Geometry: final body of the model. Coordinates: model frame, mm. Face numbers are marked on the shaded views. A direction names the side the tool comes from. Coordinates: 2 decimals unless noted, no trailing zeros. Order: outer loops, then holes, each group sorted by start corner. A loop starts at its lowest first (then second) coordinate and runs counter-clockwise, first axis right, second up. Notation, with made-up numbers: M -38.75,-17 L -0.75,-17 A25 ccw -0.75,5 Z; hole C 19,-24.5 d10. An arc over 180 degrees is marked long. Use CSV: the item, a comma, the result in double quotes. Start each with the question number.
Q1. Access query for the marked faces 4 and 5. Directions: +Z, -Z, +X, -X, +Y, -Y. A direction counts if a zero-diameter tool reaches every point of the face in a straight line with its end or side. Return the directions, or none.
Q2. Section query B-B, the plane x = 0. Output: boundary loops of the cut face in (y, z).
Q3. Section query A-A, the plane x = 28.5. Output: boundary loops of the cut face in (y, z).
Q4. First-contact query: P1, Ø12.5, axis at x = 10, z = 3, coming from the -Y side; P2, Ø12.5, axis at x = 0, z = 0, coming from the -Y side; P3, Ø1, axis at y = 7, z = 6.5, coming from the -X side; P4, Ø5, axis at x = 0, z = 0, coming from the -Y side. Flat tips, straight axial feed; report the tip coordinate or a pass-through.
Q5. Ray query, probe 1 along Y at (x, z) = (9, -11.25); probe 2 along X at (y, z) = (-23.35, 0); probe 3 along Z at (x, y) = (0, -21.3). Return the intervals inside material, ascending.
Q6. Mould query, pull axis Y, two halves, no side actions, for the marked faces 1, 2 and 3. Classes: +Y half, -Y half, draft (parallel to the pull), parting line (faces both ways), or undercut.
Q7. Section query C-C, the plane z = 6.5. Output: boundary loops of the cut face in (x, y), and give its area (3 significant figures).
Q8. Section query D-D, the plane x = 46. Output: boundary loops of the cut face in (y, z), and give its area (3 significant figures).
from build123d import *

# Parameters (mm, degrees)
CYLINDER018_R          = 4.1
CYLINDER018_DEPTH      = 10
CYLINDER018_ROLL_ANGLE = 90
CYLINDER016_R          = 10.55
CYLINDER016_DEPTH      = 10
CYLINDER016_ROLL_ANGLE = 90
PAD005_DEPTH           = 25
FILLET008_R            = 12.4


with BuildPart() as cilindro018:
    # Cylinder018 → Cylinder018 (new body)
    with BuildSketch(Plane.XY):
        Circle(CYLINDER018_R)
    extrude(amount=CYLINDER018_DEPTH)


with BuildPart() as cilindro018_1:
    # Cylinder018 roll: moved
    add(cilindro018.part.rotate(Axis((0, 0, 0), (1, 0, 0)), CYLINDER018_ROLL_ANGLE))


with BuildPart() as cilindro018_2:
    # Cylinder018 placement: moved
    add(cilindro018_1.part.moved(Location((0, -14, 0))))


with BuildPart() as obj1:
    # Cylinder016 → Cylinder016 (new body)
    with BuildSketch(Plane.XY):
        Circle(CYLINDER016_R)
    extrude(amount=CYLINDER016_DEPTH)


with BuildPart() as obj1_1:
    # Cylinder016 roll: moved
    add(obj1.part.rotate(Axis((0, 0, 0), (1, 0, 0)), CYLINDER016_ROLL_ANGLE))


with BuildPart() as obj1_2:
    # Cylinder016 placement: moved
    add(obj1_1.part.moved(Location((0, -22.5, 0))))

    # Fusion002: union Cilindro018
    add(cilindro018_2.part)


with BuildPart() as cut023004:
    # Sketch005 → Pad005 (new body)
    with BuildSketch(Plane(origin=(0, 0, 12.5), x_dir=(-1, 0, 0), z_dir=(0, 0, -1))):
        with BuildLine():
            Line((-59.749396, 29.9083), (-59.749396, -25.0917))
            Line((-59.749396, -25.0917), (15.250604, -25.0917))
            Line((15.250604, -25.0917), (15.250604, -20.0917))
            Line((15.250604, -20.0917), (-44.749396, -20.0917))
            ThreePointArc((-54.749396, -10.0917), (-51.820464, -17.162768), (-44.749396, -20.0917))
            Line((-54.749396, -10.0917), (-54.749396, 14.9083))
            ThreePointArc((-44.749396, 24.9083), (-51.820464, 21.979368), (-54.749396, 14.9083))
            Line((-44.749396, 24.9083), (15.250604, 24.9083))
            Line((15.250604, 24.9083), (15.250604, 29.9083))
            Line((15.250604, 29.9083), (-59.749396, 29.9083))
        make_face()
    extrude(amount=PAD005_DEPTH)

    # Fillet008
    fillet008_edges = [cut023004.edges().sort_by_distance(p)[0] for p in [
        (-15.250604, 27.4083, 12.5),
        (-15.250604, 27.4083, -12.5),
        (-15.250604, -22.5917, 12.5),
        (-15.250604, -22.5917, -12.5),
    ]]
    fillet(fillet008_edges, radius=FILLET008_R)

    # Cut023004: cut obj1
    add(obj1_2.part, mode=Mode.SUBTRACT)


solid = cut023004.part
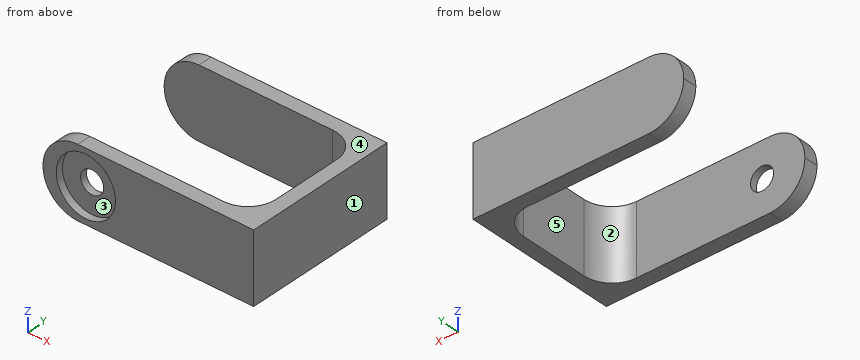
Responses:
1,face 4,"+Z, +X, -X, +Y, -Y"
1,face 5,"+Z, -Z, -X"
2,outline,"M -25.09,-12.5 L -20.09,-12.5 L -20.09,-4.1 L -22.5,-4.1 L -22.5,-10.55 L -25.09,-10.55 Z; M -25.09,10.55 L -22.5,10.55 L -22.5,4.1 L -20.09,4.1 L -20.09,12.5 L -25.09,12.5 Z; M 24.91,-12.5 L 29.91,-12.5 L 29.91,12.5 L 24.91,12.5 Z"
3,outline,"M -25.09,-12.5 L -20.09,-12.5 L -20.09,12.5 L -25.09,12.5 Z; M 24.91,-12.5 L 29.91,-12.5 L 29.91,12.5 L 24.91,12.5 Z"
4,P1,"stops at y = -25.09"
4,P2,"stops at y = -22.5"
4,P3,"stops at x = 54.75"
4,P4,"stops at y = 24.91"
5,probe 1,"y = -25.09 to -20.09, 24.91 to 29.91"
5,probe 2,"x = -15.25 to -10.55, 10.55 to 59.75"
5,probe 3,"z = -12.5 to -4.1, 4.1 to 12.5"
6,face 1,"draft"
6,face 2,"undercut"
6,face 3,"-Y half"
7,outline,"M -13.47,-25.09 L -8.31,-25.09 L -8.31,-22.5 L 8.31,-22.5 L 8.31,-25.09 L 59.75,-25.09 L 59.75,29.91 L -13.47,29.91 L -13.47,24.91 L 44.75,24.91 A10 cw 54.75,14.91 L 54.75,-10.09 A10 cw 44.75,-20.09 L -13.47,-20.09 Z"
7,area,"957 mm²"
8,outline,"M -25.09,-12.5 L -20.01,-12.5 L -20.01,12.5 L -25.09,12.5 Z; M 24.83,-12.5 L 29.91,-12.5 L 29.91,12.5 L 24.83,12.5 Z"
8,area,"254 mm²"
